Design review of the part shown in the three views and the two pictorial views. Dimensions are in mm from the part's minimum x, y and z. A direction names the side the tool comes from. Give positions to 0.01 mm unless a question says otherwise; leave off trailing zeros. Order: outer loops, then holes, each group sorted by start corner. A loop starts at its lowest first (then second) coordinate and runs counter-clockwise, first axis right, second up.
Item 1: Machinability: for the marked faces 1, 2, 3 and 4, which of the approach directions +Z, -Z, +X, -X, +Y, -Y give a long, thin tool a straight path to every point of the face, cutting with its end or side? Answer none if there is none.
Item 2: Consider section A-A (y = 15). Give the boundary of the cut face in (x, z), plus the area to 3 significant figures.
Item 3: For probe 1 along Z at (x, y) = (22, 29.5); probe 2 along Y at (x, z) = (26, 96.5); probe 3 along Z at (x, y) = (25.25, 45), list the stretches that pass through material, from the lowest coordinate up.
Item 4: Consider section D-D (z = 23.5). Give the boundary of the cut face in (x, y).
Item 5: For P1, Ø8, axis at x = 13, y = 52, coming from the +Z side; P2, Ø4, axis at x = 9, z = 54.5, coming from the -Y side; P3, Ø2, axis at x = 17.5, y = 58.5, coming from the -Z side; P4, Ø10, axis at x = 5.5, z = 59.5, coming from the -Y side, all flat-tipped, find the tip position at first contact; note any pin that passes through.
Item 6: Consider section B-B (z = 71). Give the boundary of the cut face in (x, y), plus the area to 3 significant figures.
Item 7: Consider section C-C (x = 5.75). Give the boundary of the cut face in (y, z), plus the area to 3 significant figures.
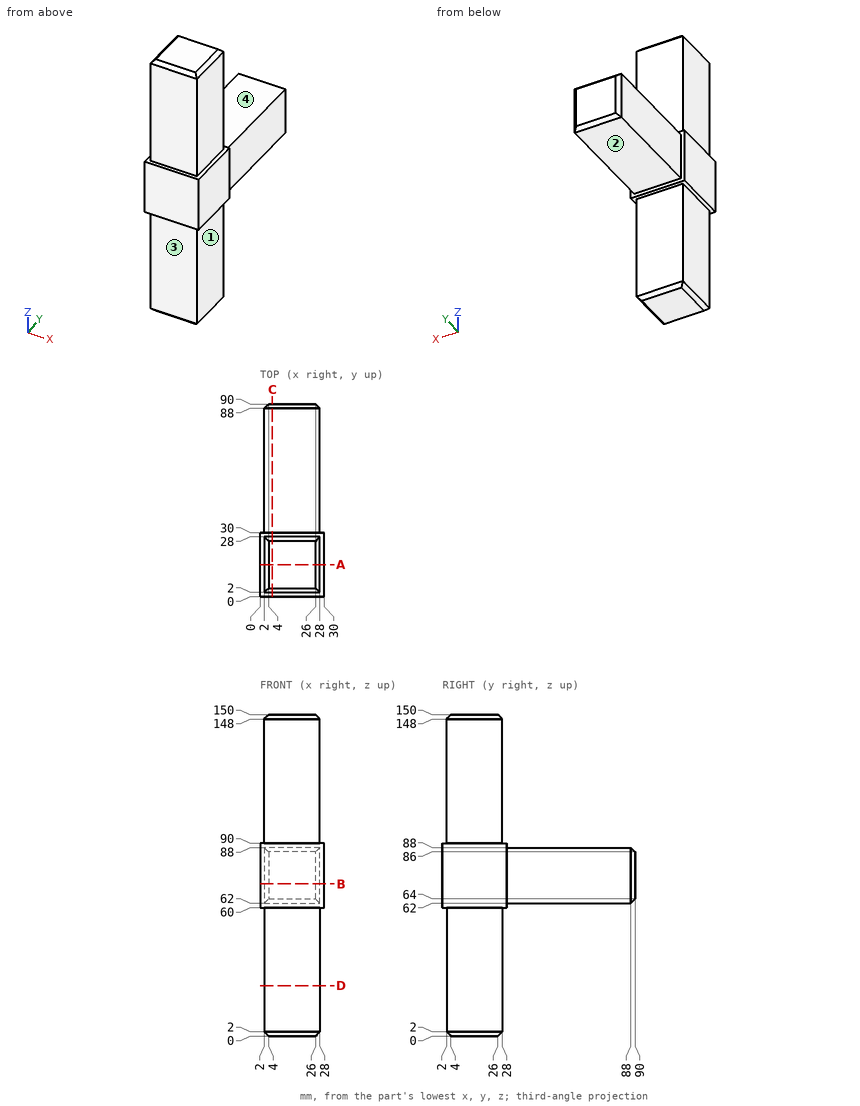
Resolved:
1. face 1: -Z, +X, +Y, -Y
1. face 2: -Z, +X, -X, +Y
1. face 3: -Z, +X, -X, -Y
1. face 4: +Z, +X, -X, +Y
2. outline: (0, 60) - (2, 60) - (2, 2) - (4, 0) - (26, 0) - (28, 2) - (28, 60) - (30, 60) - (30, 90) - (28, 90) - (28, 148) - (26, 150) - (4, 150) - (2, 148) - (2, 90) - (0, 90) - close
2. area: 4,010 mm2
3. probe 1: z = 60 to 90
3. probe 2: y = 2 to 28
3. probe 3: z = 62 to 88
4. outline: (2, 2) - (28, 2) - (28, 28) - (2, 28) - close
5. P1: stops at z = 88
5. P2: stops at y = 2
5. P3: stops at z = 62
5. P4: stops at y = 0
6. outline: (0, 0) - (30, 0) - (30, 30) - (28, 30) - (28, 88) - (26, 90) - (4, 90) - (2, 88) - (2, 30) - (0, 30) - close
6. area: 2,460 mm2
7. outline: (0, 60) - (2, 60) - (2, 2) - (4, 0) - (26, 0) - (28, 2) - (28, 60) - (30, 60) - (30, 62) - (88, 62) - (90, 64) - (90, 86) - (88, 88) - (30, 88) - (30, 90) - (28, 90) - (28, 148) - (26, 150) - (4, 150) - (2, 148) - (2, 90) - (0, 90) - close
7. area: 5,570 mm2
